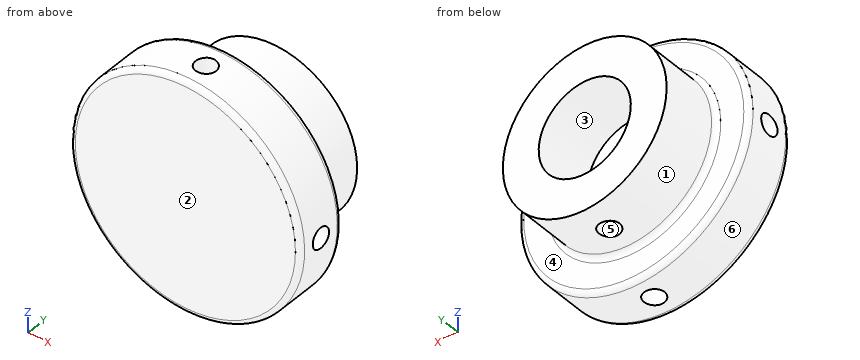
from build123d import *

# Parameters (mm, degrees)
SKETCH1_R           = 32
BOSS_EXTRUDE1_DEPTH = 24
BOSS_EXTRUDE2_START = -20
SKETCH1_4_R         = 45
SKETCH1_4_R_2       = 32
BOSS_EXTRUDE2_DEPTH = 20
SKETCH2_R           = 18
CUT_EXTRUDE1_DEPTH  = 24
CUT_EXTRUDE2_START  = -14
SKETCH3_R           = 4
CUT_EXTRUDE2_DEPTH  = 55.014704293
CIRPATTERN1_COUNT   = 4
SKETCH4_R           = 4
CUT_EXTRUDE3_DEPTH  = 69.014704425
FILLET1_R           = 2


with BuildPart() as part:
    # Sketch1 → Boss-Extrude1 (new body)
    with BuildSketch(Plane(origin=(0, 0, 0), x_dir=(1, 0, 0), z_dir=(0, 1, 0))):
        with Locations(Location((0, 0, 0), (0, 0, 270))):
            Circle(SKETCH1_R)
    extrude(amount=BOSS_EXTRUDE1_DEPTH)

    # Sketch1<4> → Boss-Extrude2 (add)
    # profile 1 of 2: a face of its own
    with BuildSketch(Plane(origin=(0, 0, 0), x_dir=(1, 0, 0), z_dir=(0, 1, 0)).offset(BOSS_EXTRUDE2_START)):
        with Locations(Location((0, 0, 0), (0, 0, 270))):
            Circle(SKETCH1_4_R)
        with Locations(Location((0, 0, 0), (0, 0, 270))):
            Circle(SKETCH1_4_R_2, mode=Mode.SUBTRACT)
    # profile 2 of 2: a face of its own
    with BuildSketch(Plane(origin=(0, 0, 0), x_dir=(1, 0, 0), z_dir=(0, 1, 0)).offset(BOSS_EXTRUDE2_START)):
        with Locations(Location((0, 0, 0), (0, 0, 270))):
            Circle(SKETCH1_4_R_2)
    extrude(amount=BOSS_EXTRUDE2_DEPTH)

    # Sketch2 → Cut-Extrude1 (cut)
    with BuildSketch(Plane(origin=(0, 24, 0), x_dir=(1, 0, 0), z_dir=(0, 1, 0))):
        with Locations(Location((0, 0, 0), (0, 0, 270))):
            Circle(SKETCH2_R)
    extrude(amount=-CUT_EXTRUDE1_DEPTH, mode=Mode.SUBTRACT)

    # Sketch3 → Cut-Extrude2 (cut, through all)
    with BuildSketch(Plane.XY.offset(CUT_EXTRUDE2_START)):
        with Locations((0, -10)):
            Circle(SKETCH3_R)
    cut_extrude2 = extrude(amount=-CUT_EXTRUDE2_DEPTH, mode=Mode.SUBTRACT)

    # CirPattern1: Cut-Extrude2 ×4 about axis
    cirpattern1_axis = Axis((0, 0, 0), (0, 1, 0))
    for i in range(1, CIRPATTERN1_COUNT):
        add(cut_extrude2.rotate(cirpattern1_axis, i * 360 / CIRPATTERN1_COUNT), mode=Mode.SUBTRACT)

    # Sketch4 → Cut-Extrude3 (cut, through all)
    with BuildSketch(Plane.XY):
        with Locations((0, 12)):
            Circle(SKETCH4_R)
    extrude(amount=-CUT_EXTRUDE3_DEPTH, mode=Mode.SUBTRACT)

    # Fillet1
    fillet1_edges = [part.edges().sort_by_distance(p)[0] for p in [
        (0, 0, -32),
        (0, -20, -45),
        (0, 0, -45),
    ]]
    fillet(fillet1_edges, radius=FILLET1_R)


solid = part.part
Part model, mm, in its own coordinate system. Face numbers are marked on the shaded views. A direction names the side the tool comes from. Coordinates: 2 decimals unless noted, no trailing zeros. Order: outer loops, then holes, each group sorted by start corner. A loop starts at its lowest first (then second) coordinate and runs counter-clockwise, first axis right, second up. Notation, with made-up numbers: M 48.25,62.5 L 60.25,62.5 A19 cw 60.25,77.5 Z; hole C 87.5,45.5 d11. An arc over 180 degrees is marked long. Use a Markdown table: item, result.
(1) Flat gauge pins, fed straight in: pin 1 (2 mm diameter, centred on x = -11.5, y = 4.5, fed in from -Z); pin 2 (6.5 mm diameter, centred on y = -10, z = 0, fed in from -X); pin 3 (9 mm diameter, centred on x = -0.5, y = -9, fed in from +Z); pin 4 (1.5 mm diameter, centred on y = -13, z = -10, fed in from -X). Where does each tip first touch, or does it go through?
A:
| item | result |
|---|---|
| pin 1 | stops at z = -30.23 |
| pin 2 | stops at x = -14 |
| pin 3 | stops at z = 45 |
| pin 4 | stops at x = -44.04 |
(2) Cut at B-B on y = -10. Write the cut outline in (x, z), then the cut area to 3 significant figures.
A:
| item | result |
|---|---|
| outline | M -44.82,-4 A45 ccw -4,-44.82 L -4,-14 L 4,-14 L 4,-44.82 A45 ccw 44.82,-4 L 14,-4 L 14,4 L 44.82,4 A45 ccw 4,44.82 L 4,14 L -4,14 L -4,44.82 A45 ccw -44.82,4 L -14,4 L -14,-4 Z |
| area | 5,370 mm^2 |
(3) Cut at C-C on z = -22.5. State how many separate pieces and enclosed holes the cut face has, then the cut area to 3 significant figures.
A:
| item | result |
|---|---|
| separate pieces | 1 |
| enclosed holes | 2 |
| area | 2,550 mm^2 |
(4) Pull direction X, two halves, no side cores. Call the marked faces 1, 2 and 3: released by +X, released by -X, zero draft, split by the parting line, or undercut.
A:
| item | result |
|---|---|
| face 1 | split by the parting line |
| face 2 | zero draft |
| face 3 | undercut |
(5) Tool access for the marked faces 4, 5 and 6: list every direction of +Z, -Z, +X, -X, +Y, -Y with a clear straight run to the whole face (end or side of a thin tool).
A:
| item | result |
|---|---|
| face 4 | +Y |
| face 5 | -Z |
| face 6 | +Y, -Y |
(6) Probe L1, parallel to Y at x = 0, z = 22; L2, parallel to Z at x = 0, y = 5. List the from-to ranges inside material, lowest first.
A:
| item | result |
|---|---|
| L1 | y = -20 to -14, -6 to 24 |
| L2 | z = -32 to -18, 18 to 32 |
(7) Cut at A-A on z = 0. Write the cut outline in (x, y).
A:
| item | result |
|---|---|
| outline | M -45,-18 A2 ccw -43,-20 L 43,-20 A2 ccw 45,-18 L 45,-14 L 14,-14 L 14,-6 L 45,-6 L 45,-2 A2 ccw 43,0 L 34,0 A2 cw 32,2 L 32,24 L 18,24 L 18,0 L -18,0 L -18,24 L -32,24 L -32,2 A2 cw -34,0 L -43,0 A2 ccw -45,-2 L -45,-6 L -14,-6 L -14,-14 L -45,-14 Z |
(8) Cut at D-D on y = 12. Write the cut outline in (x, z).
A:
| item | result |
|---|---|
| outline | M -4,-31.75 L -4,-17.55 A18 cw long 4,-17.55 L 4,-31.75 A32 ccw long Z |
